Geometry check sheet. Reference: drawing and pictorial views, mm from the part's lowest x, y, z. A direction names the side the tool comes from. Give positions to 0.01 mm unless a question says otherwise; leave off trailing zeros. Write each loop counter-clockwise with the first axis right and the second up, starting at its lowest first coordinate (ties: lowest second). Pieces come first, ordered by that corner, then holes. Notation, with made-up numbers: (-38.75, -9.75) -> (20.25, -9.75) arc R18 ccw to (20.25, 4.25) -> close; hole circle Ø2 at (12.25, 86.5). An arc over 180 degrees is marked (long way). Use a Markdown table: item, result. Add a question column.
1. Scan lines: probe 1 along X at (y, z) = (4, 5) (1 decimal); probe 2 along X at (y, z) = (4, 6.5) (1 decimal); probe 3 along X at (y, z) = (6.25, 4.25) (1 decimal). Record each from-to range of solid material in increasing order. Write a range as [from, to].
2. Set-up check for the marked faces 1, 2, 3 and 4: record each of +Z, -Z, +X, -X, +Y, -Y from which the full face is reachable in a straight line by a thin tool's end or side.
3. Cross-section at B-B (z = 5.75). Enter the section's corners in (x, y) (1 decimal).
4. Release check for a two-part mould opening along Z. For the marked faces 5, 6 and 7 record: released by +Z, released by -Z, zero draft, split by the parting line, or undercut.
5. Cross-section at D-D (x = 13.5). Enter the section's corners in (y, z), then the cut area to 3 significant figures.
6. Cross-section at A-A (x = 22). Enter the section's corners in (y, z).
7. Gauge pin test, flat ends, axial feed: P1, Ø4, axis at y = 3.5, z = 6.5, coming from the +X side; P2, Ø4, axis at x = 14, y = 5.5, coming from the +Z side; P3, Ø4, axis at y = 2, z = 1, coming from the -X side; P4, Ø1.7, axis at x = 22, z = 3.5, coming from the +Y side. Record the tip position at first contact, or that the pin passes through.
8. Cross-section at C-C (y = 4.5). Enter the section's corners in (x, z) (1 decimal), then the cut area to 3 significant figures.
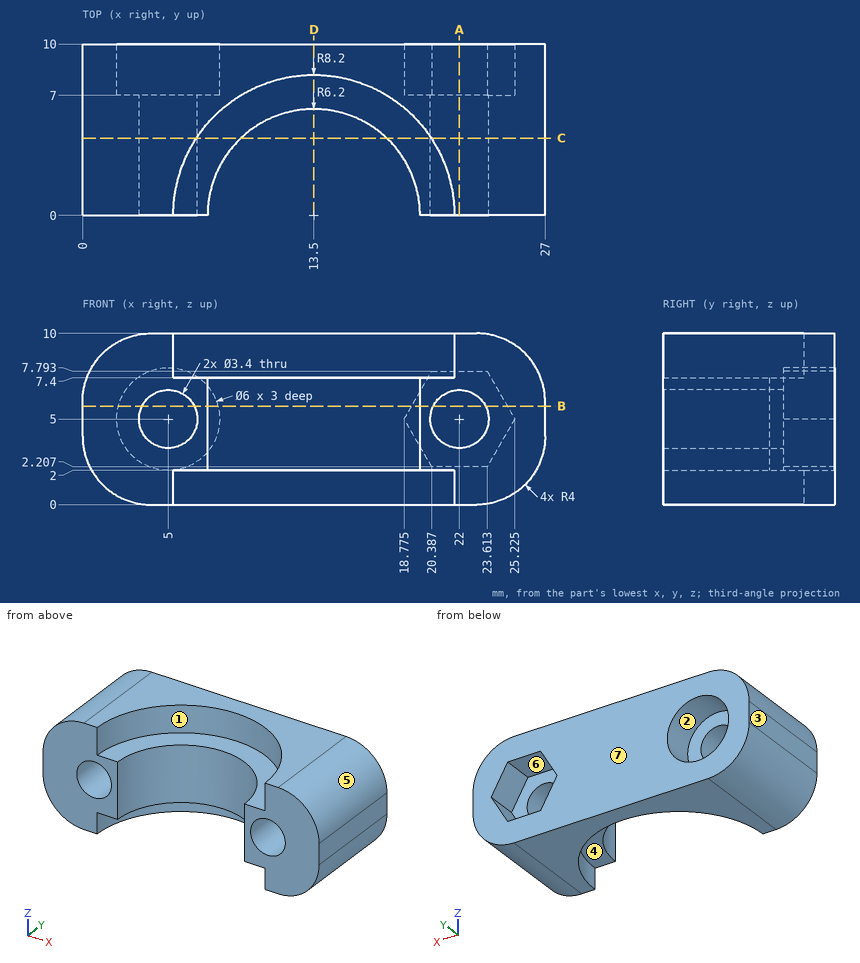
Worked answers:
| question | item | result |
|---|---|---|
| 1 | probe 1 | x = [0, 3.3], [6.7, 8.8], [18.2, 20.3], [23.7, 27] |
| 1 | probe 2 | x = [0, 4.2], [5.8, 8.8], [18.2, 21.2], [22.8, 27] |
| 1 | probe 3 | x = [0, 3.5], [6.5, 20.5], [23.5, 27] |
| 2 | face 1 | +Z, -Y |
| 2 | face 2 | +Y |
| 2 | face 3 | +Z, -Z, -X, +Y, -Y |
| 2 | face 4 | -Z, -Y |
| 3 | outline | (0, 0) -> (3.5, 0) -> (3.5, 7) -> (2.1, 7) -> (2.1, 10) -> (0, 10) -> close; (6.5, 0) -> (7.3, 0) arc R6.2 cw to (19.7, 0) -> (20.5, 0) -> (20.5, 7) -> (19.2, 7) -> (19.2, 10) -> (7.9, 10) -> (7.9, 7) -> (6.5, 7) -> close; (23.5, 0) -> (27, 0) -> (27, 10) -> (24.8, 10) -> (24.8, 7) -> (23.5, 7) -> close |
| 4 | face 5 | released by +Z |
| 4 | face 6 | undercut |
| 4 | face 7 | zero draft |
| 5 | outline | (6.2, 2) -> (8.2, 2) -> (8.2, 0) -> (10, 0) -> (10, 10) -> (8.2, 10) -> (8.2, 7.4) -> (6.2, 7.4) -> close |
| 5 | area | 28.8 mm² |
| 6 | outline | (0, 0) -> (10, 0) -> (10, 2.21) -> (7, 2.21) -> (7, 3.3) -> (0, 3.3) -> close; (0, 6.7) -> (7, 6.7) -> (7, 7.79) -> (10, 7.79) -> (10, 10) -> (0, 10) -> close |
| 7 | P1 | stops at x = 27 |
| 7 | P2 | stops at z = 7.4 |
| 7 | P3 | stops at x = 0.13 |
| 7 | P4 | stops at y = 7 |
| 8 | outline | (0, 4) arc R4 ccw to (4, 0) -> (6.6, 0) -> (6.6, 2) -> (9.2, 2) -> (9.2, 7.4) -> (6.6, 7.4) -> (6.6, 10) -> (4, 10) arc R4 ccw to (0, 6) -> close; (17.8, 2) -> (20.4, 2) -> (20.4, 0) -> (23, 0) arc R4 ccw to (27, 4) -> (27, 6) arc R4 ccw to (23, 10) -> (20.4, 10) -> (20.4, 7.4) -> (17.8, 7.4) -> close; hole circle Ø3.4 at (5, 5); hole circle Ø3.4 at (22, 5) |
| 8 | area | 129 mm² |
